Design review of the part built by this model. Coordinates are the model's own, in mm. A direction names the side the tool comes from. Round coordinates to 2 decimals unless told otherwise and drop trailing zeros. Loops run counter-clockwise (first coordinate to the right, second up) from the corner with the lowest first, then second, coordinate; pieces in that order, holes last. Notation, with made-up numbers: M 80,69 L 92,69 A4 cw 92,75 Z; hole C 76.5,43 d1. An arc over 180 degrees is marked long. Use a Markdown table: item, result.
Autodesk Inventor part; units mm, degrees
ref_plane "YZ Plane" through (0, 0, 0) normal (1, 0, 0) x (0, 1, 0)
ref_plane "XZ Plane" through (0, 0, 0) normal (0, 1, 0) x (-1, 0, 0)
ref_plane "XY Plane" through (0, 0, 0) normal (0, 0, 1) x (1, 0, 0)
sketch "Sketch1" plane through (0, 0, 0) normal (0, 1, 0) x (-1, 0, 0)
  circle A0 centre (0, 0) radius 90
  line L0 (21.15, 21.15) -> (-21.15, 21.15) construction
  line L1 (-21.15, 21.15) -> (-21.15, -21.15) construction
  line L2 (-21.15, -21.15) -> (21.15, -21.15) construction
  line L3 (21.15, -21.15) -> (21.15, 21.15) construction
  line L4 (21.15, 21.15) -> (-21.15, -21.15) construction
  line L5 (-21.15, 21.15) -> (21.15, -21.15) construction
  circle A1 centre (0, 0) radius 10
  dimension "d0" = 180
  dimension "d1" = 42.3
  dimension "d2" = 42.3
  dimension "d3" = 20
extrude "Extrusion1" add sketch "Sketch1" along normal blind 10
sketch "Sketch2" plane through (0, 0, 0) normal (0, -1, 0) x (1, 0, 0)
  circle A0 centre (0, 0) radius 15
  circle A1 centre (0, 0) radius 10
  dimension "d6" = 30
  dimension "d7" = 20
extrude "Extrusion2" add sketch "Sketch2" along normal blind 3
sketch "Sketch3" plane through (0, -3, 0) normal (0, -1, 0) x (1, 0, 0)
  circle A0 centre (0, 0) radius 10
  circle A1 centre (0, 0) radius 12.5
  dimension "d10" = 25
  dimension "d11" = 20
extrude "Extrusion3" add sketch "Sketch3" along normal blind 12
sketch "Sketch4" plane through (0, 10, 0) normal (0, 1, 0) x (1, 0, 0)
  line L0 (-21.15, -21.15) -> (21.15, -21.15)
  line L1 (21.15, -21.15) -> (21.15, 21.15)
  line L2 (21.15, 21.15) -> (-21.15, 21.15)
  line L3 (-21.15, 21.15) -> (-21.15, -21.15)
  line L4 (-21.15, -21.15) -> (21.15, 21.15) construction
  line L5 (21.15, -21.15) -> (-21.15, 21.15) construction
  line L6 (-15.15, -15.15) -> (15.15, -15.15)
  line L7 (15.15, -15.15) -> (15.15, 15.15)
  line L8 (15.15, 15.15) -> (-15.15, 15.15)
  line L9 (-15.15, 15.15) -> (-15.15, -15.15)
  line L10 (-15.15, -15.15) -> (15.15, 15.15) construction
  line L11 (15.15, -15.15) -> (-15.15, 15.15) construction
  point P0 (0, 0)
  dimension "d14" = 42.3
  dimension "d15" = 42.3
  dimension "d16" = 6
extrude "Extrusion4" add sketch "Sketch4" along normal blind 10
sketch "Sketch5" plane through (21.15, 10, -21.15) normal (0, 0, -1) x (-1, 0, 0)
  line L0 (11.15, 5) -> (31.15, 5) construction
  line L1 (11.15, 2.5) -> (31.15, 2.5)
  line L2 (31.15, 7.5) -> (11.15, 7.5)
  arc A0 (11.15, 7.5) -> (11.15, 2.5) centre (11.15, 5) ccw
  arc A1 (31.15, 2.5) -> (31.15, 7.5) centre (31.15, 5) ccw
  line L3 (0, 10) -> (42.3, 10)
  point P0 (21.15, -10)
  point P1 (21.15, 5)
  dimension "d19" = 5
  dimension "d20" = 20
  dimension "d21" = 2.5
extrude "Extrusion5" cut sketch "Sketch5" against normal through all
sketch "Sketch6" plane through (0, 10, 0) normal (0, 1, 0) x (1, 0, 0)
  circle A0 centre (-30, 15.5) radius 1.5
  line L0 (0, 0) -> (41.4965, 0) construction
  line L1 (0, 0) -> (0, 38.6106) construction
  circle A1 centre (30, 15.5) radius 1.5
  circle A2 centre (-30, -15.5) radius 1.5
  circle A3 centre (30, -15.5) radius 1.5
  line L2 (-9.5, 62.5) -> (9.5, 62.5) construction
  line L3 (9.5, 62.5) -> (9.5, 47.5) construction
  line L4 (9.5, 47.5) -> (-9.5, 47.5) construction
  line L5 (-9.5, 47.5) -> (-9.5, 62.5) construction
  line L6 (-9.5, 62.5) -> (9.5, 47.5) construction
  line L7 (9.5, 62.5) -> (-9.5, 47.5) construction
  circle A4 centre (-7.5, 60.5) radius 1.5
  circle A5 centre (7.5, 60.5) radius 1.5
  point P0 (0, 55)
  dimension "d24" = 3
  dimension "d25" = 30
  dimension "d26" = 15.5
  dimension "d29" = 60
  dimension "d32" = 31
  dimension "d35" = 15
  dimension "d36" = 19
  dimension "d37" = 55
  dimension "d38" = 2
  dimension "d39" = 2
  dimension "d40" = 3
extrude "Extrusion6" cut sketch "Sketch6" against normal through all
equation "\"d2\" = d1"
equation "\"d15\" = d14"
properties part number "Satellite_plate_3DPrint"
1. Take a section at C-C on z = 54. Give the boundary of the cut face in (x, y).
Check values:
| item | result |
|---|---|
| outline | M -72,0 L 72,0 L 72,10 L -72,10 Z |
2. Machinability: for faces 4 (the face through (-12.5, 14.9, -18.2)), 5 (the face through (-14.985, -1.479, -0.66)), 6 (the face through (0, 18, 21.15)), which of the approach directions +Z, -Z, +X, -X, +Y, -Y give a long, thin tool a straight path to every point of the face, cutting with its end or side? Answer none if there is none.
Check values:
| item | result |
|---|---|
| face 4 | +Z, -Z |
| face 5 | -Y |
| face 6 | +Z, +X, -X, +Y |
3. The part is to be moulded in two halves that separate along Y. For faces 1 (the face through (0, 12.5, -18)), 2 (the face through (-3.4, -3, 12.3)), 3 (the face through (-15.15, 15, 0)), say which applies: pulls with the +Y half, pulls with the -Y half, needs draft (parallel to the pull), parting line crosses it, or undercut.
Check values:
| item | result |
|---|---|
| face 1 | undercut |
| face 2 | pulls with the -Y half |
| face 3 | needs draft |
4. Take a section at B-B on y = -6. Give the boundary of the cut face in (x, z), and give its area (3 significant figures).
Check values:
| item | result |
|---|---|
| outline | C 0,0 d25; hole C 0,0 d20 |
| area | 177 mm² |
5. Insertion check: pin 1 (3 mm diameter, centred on x = 36.5, y = 6, fed in from -Z); pin 2 (23 mm diameter, centred on x = 0, z = 0, fed in from +Y); pin 3 (18 mm diameter, centred on x = 0, z = 0, fed in from +Y); pin 4 (5 mm diameter, centred on x = -56, z = -26.5, fed in from -Y). Each pin has a flat end and moves straight along its axis. Give the tip position at first contact, or say it passes through.
Check values:
| item | result |
|---|---|
| pin 1 | stops at z = -82.92 |
| pin 2 | stops at y = 10 |
| pin 3 | passes through |
| pin 4 | stops at y = 0 |
6. Take a section at D-D on x = -35. Give the boundary of the cut face in (y, z).
Check values:
| item | result |
|---|---|
| outline | M 0,-82.92 L 10,-82.92 L 10,82.92 L 0,82.92 Z |
7. Wall thickness on line 1 along Z through (x, y) = (0, -1); line 2 along Z through (x, y) = (0, 4); line 3 along X through (y, z) = (11.5, 11): over which ranges is each line inside the solid? List them lowest first. Write a range as from..to.
Check values:
| item | result |
|---|---|
| line 1 | z = -15..-10, 10..15 |
| line 2 | z = -90..-10, 10..90 |
| line 3 | x = -21.15..-15.15, 15.15..21.15 |
8. Take a section at A-A on y = 4. Give the boundary of the cut face in (x, z), and give its area (3 significant figures).
Check values:
| item | result |
|---|---|
| outline | C 0,0 d180; hole C -30,-15.5 d3; hole C -30,15.5 d3; hole C 0,0 d20; hole C -7.5,-60.5 d3; hole C 7.5,-60.5 d3; hole C 30,-15.5 d3; hole C 30,15.5 d3 |
| area | 25,100 mm² |
